```python
from build123d import *

# Parameters (mm, degrees)
ESQUISSE1_W             = 45
ESQUISSE1_H             = 8
ESQUISSE1_R             = 1.5
BOSS_EXTRU_1_DEPTH      = 3
ESQUISSE2_W             = 45
ESQUISSE2_H             = 3
BOSS_EXTRU_2_DEPTH      = 20
ESQUISSE3_R             = 1.75
ENL_V_MAT_EXTRU_1_DEPTH = 20


with BuildPart() as part:
    # Esquisse1 → Boss.-Extru.1 (new body)
    with BuildSketch(Plane(origin=(0, 0, 0), x_dir=(1, 0, 0), z_dir=(0, 1, 0))):
        with Locations((1.515789474, 0.846662995)):
            Rectangle(ESQUISSE1_W, ESQUISSE1_H)
        with Locations(Location((19.515789474, 0, 0), (0, 0, 270))):
            Circle(ESQUISSE1_R, mode=Mode.SUBTRACT)
        with Locations(Location((-16.484210526, 0, 0), (0, 0, 270))):
            Circle(ESQUISSE1_R, mode=Mode.SUBTRACT)
    extrude(amount=BOSS_EXTRU_1_DEPTH)

    # Esquisse2 → Boss.-Extru.2 (add)
    with BuildSketch(Plane(origin=(0, 3, 0), x_dir=(1, 0, 0), z_dir=(0, 1, 0))):
        with Locations((1.515789474, 3.346662995)):
            Rectangle(ESQUISSE2_W, ESQUISSE2_H)
    extrude(amount=BOSS_EXTRU_2_DEPTH)

    # Esquisse3 → Enlèv. mat.-Extru.1 (cut)
    with BuildSketch(Plane.XY.offset(-1.846662995)):
        with Locations((1.515789474, 18)):
            Circle(ESQUISSE3_R)
    extrude(amount=-ENL_V_MAT_EXTRU_1_DEPTH, mode=Mode.SUBTRACT)


solid = part.part
```
Can you work these out from the model? Positions are in its coordinate system, mm. A direction names the side the tool comes from. Coordinates: 2 decimals unless noted, no trailing zeros. Loops run counter-clockwise (first coordinate to the right, second up) from the corner with the lowest first, then second, coordinate; pieces in that order, holes last.
Item 1: Suppose I cut it at C-C (x = 0.5). Please give me the cut outline in (y, z), then the cut area to 4 significant figures.
Answers below:
outline: (0, -4.85) - (16.57, -4.85) - (16.57, -1.85) - (3, -1.85) - (3, 3.15) - (0, 3.15) - close; (19.43, -4.85) - (23, -4.85) - (23, -1.85) - (19.43, -1.85) - close
area: 75.45 mm2
Item 2: If we mould it in two halves opening along Z, with no side actions, what happens to faces 1 (the face through (1, 11, -4.847)), 2 (the face through (20.78, 1.48, 0.81)), 3 (the face through (24.016, 9, -3)), 4 (the face through (1, 1, 3.153))? For each: released by +Z, released by -Z, zero draft, split by the parting line, or undercut.
Answers below:
face 1: released by -Z
face 2: undercut
face 3: zero draft
face 4: released by +Z
Item 3: Which directions (+Z, -Z, +X, -X, +Y, -Y) give clear straight access to the entire face, cutting with the end or side of a thin tool? Please do faces 5 (the face through (1, 0, -1)), 6 (the face through (1, 13, -1.847)).
Answers below:
face 5: +Z, -Z, +X, -X, -Y
face 6: +Z, +X, -X, +Y
Item 4: Suppose I cut it at A-A (z = 0). Please give me the cut outline in (x, y), then the cut area to 3 significant figures.
Answers below:
outline: (-20.98, 0) - (-17.98, 0) - (-17.98, 3) - (-20.98, 3) - close; (-14.98, 0) - (18.02, 0) - (18.02, 3) - (-14.98, 3) - close; (21.02, 0) - (24.02, 0) - (24.02, 3) - (21.02, 3) - close
area: 117 mm2
Item 5: Please list where these lines run through material, in increasing order: L1, parallel to X at y = 1.1, z = 0; L2, parallel to Z at x = 18.5, y = 6.25; L3, parallel to Y at x = 8.5, z = -0.75.
Answers below:
L1: x = -20.98 to -17.98, -14.98 to 18.02, 21.02 to 24.02
L2: z = -4.85 to -1.85
L3: y = 0 to 3
Item 6: Suppose I cut it at B-B (y = 18). Please give me the cut outline in (x, z).
Answers below:
outline: (-20.98, -4.85) - (-0.23, -4.85) - (-0.23, -1.85) - (-20.98, -1.85) - close; (3.27, -4.85) - (24.02, -4.85) - (24.02, -1.85) - (3.27, -1.85) - close
Item 7: I'm going to push a flat-ended pin straight in: pin 1 (3 mm diameter, centred on y = 18.5, z = -0.5, fed in from -X). Where does the tip first touch, or does it pass through?
Answers below:
pin 1: stops at x = -20.98
Item 8: Suppose I cut it at D-D (x = 5). Please give me the cut outline in (y, z).
Answers below:
outline: (0, -4.85) - (23, -4.85) - (23, -1.85) - (3, -1.85) - (3, 3.15) - (0, 3.15) - close
